Autodesk Inventor part; units mm, degrees
ref_plane "YZ Plane" through (0, 0, 0) normal (1, 0, 0) x (0, 1, 0)
ref_plane "XZ Plane" through (0, 0, 0) normal (0, 1, 0) x (-1, 0, 0)
ref_plane "XY Plane" through (0, 0, 0) normal (0, 0, 1) x (1, 0, 0)
sketch "スケッチ1" plane through (0, 0, 0) normal (0, 0, 1) x (1, 0, 0)
  circle A0 centre (70, 10) radius 6.025
  circle A1 centre (70, 10) radius 9
  arc A2 (70.8604, 37.0956) -> (76.1852, 16.5379) centre (89.93, 31.0664) ccw
  arc A3 (-3.9904, -8.067) -> (76.0896, 3.373) centre (27.7113, 56.0206) ccw
  arc A4 (70.6777, 25.6489) -> (65.6559, 26.9449) centre (67.7899, 24.8363) ccw
  arc A5 (59.3301, 20.543) -> (55.2759, 7.1361) centre (70, 10) ccw
  arc A6 (57.575, -4.684) -> (61.9566, -6.7447) centre (60.5198, -4.1112) ccw
  line L0 (67.7899, 24.8363) -> (70, 10) construction
  line L1 (70, 10) -> (60.5198, -4.1112) construction
  circle A7 centre (67.7899, 24.8363) radius 1.5
  circle A8 centre (60.5198, -4.1112) radius 1.5
  line L2 (70, 10) -> (59.7573, 12.3103) construction
  circle A9 centre (59.7573, 12.3103) radius 1.5
  line L3 (59.3301, 20.543) -> (65.6559, 26.9449)
  line L4 (55.2759, 7.1361) -> (57.575, -4.684)
  point P0 (0, 0)
  point P1 (0, 0)
  dimension "d0" = 3
  dimension "d1" = 3
  dimension "d2" = 3
  dimension "d3" = 3
  dimension "d4" = 3
  dimension "d5" = 15
  dimension "d6" = 17
extrude "押し出し1" add sketch "スケッチ1" along normal blind 6
sketch "スケッチ2" plane through (0, 0, 6) normal (0, 0, 1) x (1, 0, 0)
  point P0 (0, 0)
sketch "スケッチ3" plane through (0, 0, 6) normal (0, 0, 1) x (1, 0, 0)
  line L0 (65.6559, 26.9449) -> (59.3301, 20.543)
  arc A0 (59.3301, 20.543) -> (55.2759, 7.1361) centre (70, 10) ccw
  line L1 (55.2759, 7.1361) -> (57.575, -4.684)
  arc A1 (57.575, -4.684) -> (61.9566, -6.7447) centre (60.5198, -4.1112) ccw
  arc A2 (61.9566, -6.7447) -> (76.0896, 3.373) centre (27.7113, 56.0206) ccw
  arc A3 (76.0896, 3.373) -> (76.1852, 16.5379) centre (70, 10) ccw
  arc A4 (70.6777, 25.6489) -> (76.1852, 16.5379) centre (89.93, 31.0664) ccw
  arc A5 (70.6777, 25.6489) -> (65.6559, 26.9449) centre (67.7899, 24.8363) ccw
  circle A6 centre (70, 10) radius 6.025
  circle A7 centre (59.7573, 12.3103) radius 1.5
  circle A8 centre (67.7899, 24.8363) radius 1.5
  circle A9 centre (60.5198, -4.1112) radius 1.5
  circle A10 centre (70, 10) radius 8
  line L2 (65.9307, 16.8878) -> (72.7106, 20.8933)
  line L3 (63.4649, 5.3856) -> (68.9527, -2.3863)
  point P0 (0, 0)
  dimension "d9" = 16
extrude "押し出し2" cut sketch "スケッチ3" against normal blind 3 contours A4 A3 A2 L3 A10 L2 | A10
properties part number "前足フレーム補助パーツ" material "アルミニウム 2014-T6"
Design review of the part built by this model. Coordinates are the model's own, in mm. A direction names the side the tool comes from. Coordinates: 2 decimals unless noted, no trailing zeros. Order: outer loops, then holes, each group sorted by start corner. A loop starts at its lowest first (then second) coordinate and runs counter-clockwise, first axis right, second up. Notation, with made-up numbers: (51.25, 63.5) -> (89.25, 63.5) arc R16 ccw to (89.25, 91.5) -> close; hole circle Ø3 at (-9, 7.5). An arc over 180 degrees is marked (long way). One line per item, written item: value. Start each with the question number.
Q1. Tool access review of faces 1 (the cylindrical face through (67.843, -3.154, 2.291)), 2 (the flat face through (72, 4, 3)): name each direction out of +Z, -Z, +X, -X, +Y, -Y from which nothing blocks a thin tool from reaching the whole face with its end or side.
Q2. Take a section at C-C, the plane z = 0.4. State the section outline as (x, y) points (3 decimals).
Q3. Take a section at D-D, the plane z = 3.85. State the section outline as (x, y) points (3 decimals), then the cut area to 3 significant figures.
Q4. Insertion check: pin 1 Ø3 at (y, z) = (4.5, 2) entering from +X; pin 2 Ø4 at (x, y) = (59.76, 12.31) entering from -Z; pin 3 Ø1.5 at (y, z) = (17, 1.5) entering from -X; pin 4 Ø1.5 at (y, z) = (-2.5, 1.5) entering from +X. Each pin has a flat end and moves straight along its axis. Give the tip position at first contact, or say it passes through.
Q5. For probe 1 along Y at (x, z) = (68.75, 1.8); probe 2 along X at (y, z) = (13, 1.25) (3 decimals); probe 3 along Y at (x, z) = (67, 4.4), list the stretches that pass through material, from the lowest coordinate up.
Q6. Take a section at B-B, the plane x = 60.5. State the section outline as (y, z) points.
Q7. Mouldability with a two-part tool opening along X and no side actions: class faces 3 (the cylindrical face through (68.5, 27.75, 2.96)), 4 (the cylindrical face through (79, 10, 1)), 5 (the cylindrical face through (58.567, 13.223, 2.958)) as pulls with the +X half, pulls with the -X half, needs draft (parallel to the pull), parting line crosses it, or undercut.
Q8. Take a section at A-A, the plane y = 10. State the section outline as (x, z) points (3 decimals), then the cut area to 3 significant figures.
Values follow:
1. face 1: +Z, -Z, +X, -Y
1. face 2: +Z, +X
2. outline: (55.276, 7.136) -> (57.575, -4.684) arc R3 ccw to (61.957, -6.745) arc R71.5 ccw to (76.09, 3.373) arc R9 ccw to (76.185, 16.538) arc R20 cw to (70.678, 25.649) arc R3 ccw to (65.656, 26.945) -> (59.33, 20.543) arc R15 ccw to start; hole circle Ø3 at (59.757, 12.31); hole circle Ø3 at (60.52, -4.111); hole circle Ø12.05 at (70, 10); hole circle Ø3 at (67.79, 24.836)
3. outline: (55.276, 7.136) -> (57.575, -4.684) arc R3 ccw to (61.957, -6.745) arc R71.5 ccw to (68.953, -2.386) -> (63.465, 5.386) arc R8 cw to (65.931, 16.888) -> (72.711, 20.893) arc R20 cw to (70.678, 25.649) arc R3 ccw to (65.656, 26.945) -> (59.33, 20.543) arc R15 ccw to start; hole circle Ø3 at (59.757, 12.31); hole circle Ø3 at (60.52, -4.111); hole circle Ø3 at (67.79, 24.836)
3. area: 276 mm2
4. pin 1: stops at x = 78.06
4. pin 2: stops at z = 0
4. pin 3: stops at x = 56.36
4. pin 4: stops at x = 69.84
5. probe 1: y = -2.53 to 4.11, 15.89 to 23.68, 25.99 to 27.68
5. probe 2: x = 55.303 to 58.425, 61.089 to 64.775, 75.225 to 78.485
5. probe 3: y = -3.72 to 0.38, 17.52 to 23.56, 26.11 to 27.73
6. outline: (-7.11, 0) -> (-5.61, 0) -> (-5.61, 6) -> (-7.11, 6) -> close; (-2.61, 0) -> (11.01, 0) -> (11.01, 6) -> (-2.61, 6) -> close; (13.61, 0) -> (21.73, 0) -> (21.73, 6) -> (13.61, 6) -> close
7. face 3: parting line crosses it
7. face 4: pulls with the +X half
7. face 5: undercut
8. outline: (55, 0) -> (63.975, 0) -> (63.975, 3) -> (62, 3) -> (62, 6) -> (55, 6) -> close; (76.025, 0) -> (79, 0) -> (79, 3) -> (76.025, 3) -> close
8. area: 56.9 mm2
